```python
from build123d import *

# Parameters (mm, degrees)
SKETCH1_R           = 1.5367
SKETCH1_R_2         = 1.537816199
SKETCH1_W           = 6.2611
SKETCH1_H           = 3.0861
SKETCH1_W_2         = 6.35
SKETCH1_H_2         = 12.7
SKETCH1_W_3         = 3.0861
SKETCH1_H_3         = 6.2611
BOSS_EXTRUDE5_DEPTH = 20


with BuildPart() as part:
    # Sketch1 → Boss-Extrude5 (new body)
    with BuildSketch(Plane.XY):
        with BuildLine():
            Line((0, 0), (95.25, 0))
            Line((95.25, 0), (95.25, 114.3))
            Line((95.25, 114.3), (64.625, 114.3))
            Line((64.625, 114.3), (64.625, 96.8375))
            ThreePointArc((64.625, 96.8375), (47.625, 79.8375), (30.625, 96.8375))
            Line((30.625, 96.8375), (30.625, 114.3))
            Line((30.625, 114.3), (0, 114.3))
            Line((0, 114.3), (0, 0))
        make_face()
        with Locations((84.348005256, 23.852932932)):
            Circle(SKETCH1_R, mode=Mode.SUBTRACT)
        with Locations((10.458289057, 23.852932932)):
            Circle(SKETCH1_R_2, mode=Mode.SUBTRACT)
        with Locations((6.39445, 4.80695)):
            Rectangle(SKETCH1_W, SKETCH1_H, mode=Mode.SUBTRACT)
        with Locations((47.625, 47.625)):
            Rectangle(SKETCH1_W_2, SKETCH1_H_2, mode=Mode.SUBTRACT)
        with Locations((90.44305, 6.39445)):
            Rectangle(SKETCH1_W_3, SKETCH1_H_3, mode=Mode.SUBTRACT)
        with Locations((4.80695, 107.90555)):
            Rectangle(SKETCH1_W_3, SKETCH1_H_3, mode=Mode.SUBTRACT)
        with Locations((88.85555, 109.49305)):
            Rectangle(SKETCH1_W, SKETCH1_H, mode=Mode.SUBTRACT)
    extrude(amount=BOSS_EXTRUDE5_DEPTH)


solid = part.part
```
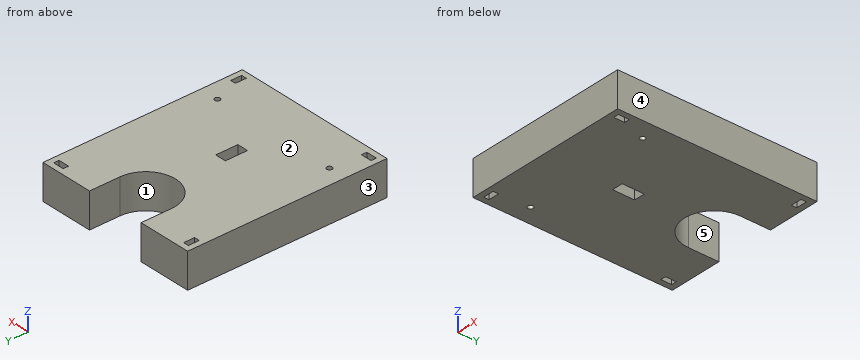
Work out the finished part from the listing and answer in its coordinate system (mm). Face numbers are marked on the shaded views. A direction names the side the tool comes from. Coordinates: 2 decimals unless noted, no trailing zeros. Loops run counter-clockwise (first coordinate to the right, second up) from the corner with the lowest first, then second, coordinate; pieces in that order, holes last. Notation, with made-up numbers: M 59.5,-12 L 99.5,-12 A22 cw 99.5,19 Z; hole C 25,-23 d2. An arc over 180 degrees is marked long. Use CSV: the item, a comma, the result in double quotes. Start each with the question number.
(1) For a pull along X with two mould halves and no side action, classify the marked faces 1, 2 and 3 as +X half, -X half, draft (parallel to the pull), parting line (faces both ways), or undercut.
(2) Consider line 1 (X direction, y = 98.5, z = 10.25) (3 decimals); line 2 (X direction, y = 47.5, z = 18.75); line 3 (Y direction, x = 11.5, z = 3). Determine where each line is inside the solid, lowest interval first.
(3) Find section D-D, the plane x = 56. Give the vertices of the cut face in (y, z), then the cut area to 3 significant figures.
(4) Find section C-C, the plane z = 8. State how many separate pieces and enclosed holes the cut face has, then the cut area to 3 significant figures.
(5) Find section B-B, the plane x = 46. Give the vertices of the cut face in (y, z) (3 decimals).
(6) For the marked faces 4 and 5, determine the directions among +Z, -Z, +X, -X, +Y, -Y from which every point of the face is accessible in a straight line to the end or side of a thin tool.
(7) Find section A-A, the plane y = 50. Give the vertices of the cut face in (x, z), then the cut area to 3 significant figures.
Recorded:
1,face 1,"undercut"
1,face 2,"draft"
1,face 3,"-X half"
2,line 1,"x = 0 to 30.625, 64.625 to 95.25"
2,line 2,"x = 0 to 44.45, 50.8 to 95.25"
2,line 3,"y = 0 to 22.72, 24.98 to 114.3"
3,outline,"M 0,0 L 82.04,0 L 82.04,20 L 0,20 Z"
3,area,"1,640 mm^2"
4,separate pieces,"1"
4,enclosed holes,"7"
4,area,"9,670 mm^2"
5,outline,"M 0,0 L 41.275,0 L 41.275,20 L 0,20 Z; M 53.975,0 L 79.915,0 L 79.915,20 L 53.975,20 Z"
6,face 4,"+Z, -Z, +X, +Y, -Y"
6,face 5,"+Z, -Z, +Y"
7,outline,"M 0,0 L 44.45,0 L 44.45,20 L 0,20 Z; M 50.8,0 L 95.25,0 L 95.25,20 L 50.8,20 Z"
7,area,"1,780 mm^2"
